Can you work these out from the model? Positions are in its coordinate system, mm. A direction names the side the tool comes from. Round coordinates to 2 decimals unless told otherwise and drop trailing zeros. Write each loop counter-clockwise with the first axis right and the second up, starting at its lowest first coordinate (ties: lowest second). Pieces come first, ordered by that corner, then holes. Notation, with made-up numbers: (44.5, 82.25) - (103.5, 82.25) arc R27 ccw to (103.5, 116.25) - close; hole circle Ø4 at (-33, 84.5). An arc over 180 degrees is marked (long way). One line per item, written item: value. Start each with the question number.
(1) On a 3-axis mill with a long thin cutter (end or side, diameter ignored), from which of +Z, -Z, +X, -X, +Y, -Y can I reach the whole of each face in a straight line? I mean faces 1 (the face through (3, 78.012, 3)), 2 (the face through (3, 135.162, 3)), 3 (the face through (168, 78.012, 3)). Say none if no direction works.
(2) I want a section at A-A on z = 2. Give the number of separate pieces and of enclosed holes in the cut face, plus the area to 3 significant figures.
(3) I want a section at C-C on y = 71. List the corners of the cut face in (x, z) for me, plus the area to 3 significant figures.
(4) If I drill on L1, parallel to X at y = 128.5, z = 1.5; L2, parallel to X at y = 117.5, z = 1; L3, parallel to Y at x = 203, z = 2, over which ranges is the centre line in solid material (lowest first)? Write a range as from..to.
(5) I want a section at B-B on x = 142. List the corners of the cut face in (y, z) for me, plus the area to 3 significant figures.
(6) I'm going to push flat-ended pins straight in: pin 1 Ø1.5 at (x, z) = (180.5, 2) entering from -Y; pin 2 Ø3 at (x, z) = (6.5, 3) entering from +Y. Where does each tip first touch, or does it pass through?
Autodesk Inventor part; units mm, degrees
ref_plane "YZ Plane" through (0, 0, 0) normal (1, 0, 0) x (0, 1, 0)
ref_plane "XZ Plane" through (0, 0, 0) normal (0, 1, 0) x (-1, 0, 0)
ref_plane "XY Plane" through (0, 0, 0) normal (0, 0, 1) x (1, 0, 0)
sketch "Sketch1" plane through (0, 0, 0) normal (0, 0, 1) x (1, 0, 0)
  line L0 (0, 78.0122) -> (0, 82.508)
  line L1 (-6.35, 82.508) -> (-6.35, 78.0122)
  line L2 (-6.35, 78.0122) -> (0, 78.0122)
  line L3 (222.25, 130.6664) -> (222.25, 135.1622)
  line L4 (215.9, 135.1622) -> (222.25, 135.1622)
  line L5 (215.9, 135.1622) -> (215.9, 130.6664)
  line L6 (222.25, 78.0122) -> (222.25, 135.1622)
  line L7 (-6.35, 135.1622) -> (-6.35, 78.0122)
  arc A0 (65.1726, 108.6235) -> (63.7223, 104.0872) centre (63.7223, 106.5872) ccw
  line L8 (222.25, 135.1622) -> (108.3945, 135.1622)
  line L9 (19.05, 135.1622) -> (-6.35, 135.1622)
  line L10 (-6.35, 78.0122) -> (19.05, 78.0122)
  line L11 (108.3945, 78.0122) -> (222.25, 78.0122)
  arc A1 (108.3945, 135.1622) -> (19.05, 135.1622) centre (63.7223, 106.5872) ccw
  arc A2 (19.05, 78.0122) -> (108.3945, 78.0122) centre (63.7223, 106.5872) ccw
  line L12 (215.9, 130.6664) -> (222.25, 130.6664)
  line L13 (0, 82.508) -> (-6.35, 82.508)
  point P0 (0, 0)
  dimension "d19" = 57.15
  dimension "d20" = 57.15
  dimension "d21" = 228.6
  dimension "d22" = 228.6
  dimension "d23" = 25.4
  dimension "d24" = 25.4
  dimension "d25" = 113.8555
  dimension "d26" = 113.8555
extrude "Extrusion1" add sketch "Sketch1" along normal blind 6.35
extrude "Extrusion2" [suppressed]
sketch "Sketch3" plane through (0, 0, 0) normal (0, 0, -1) x (-1, 0, 0)
  line L0 (6.35, 135.1622) -> (6.35, 78.0122) construction
  line L1 (-222.25, 135.1622) -> (-108.3945, 135.1622) construction
  line L2 (-222.25, 78.0122) -> (-222.25, 135.1622) construction
  line L3 (-108.3945, 78.0122) -> (-222.25, 78.0122) construction
  line L4 (-215.9, 135.1622) -> (-215.9, 130.6664) construction
  line L5 (-217.6131, 96.5879) -> (-200.4173, 96.5879) construction
  line L6 (-200.4173, 90.2379) -> (-217.6131, 90.2379) construction
  line L7 (-217.6131, 90.2379) -> (-217.6131, 96.5879) construction
  line L8 (-217.6131, 121.9879) -> (-200.4173, 121.9879) construction
  line L9 (-200.4173, 115.6379) -> (-217.6131, 115.6379) construction
  line L10 (-217.6131, 115.6379) -> (-217.6131, 121.9879) construction
  circle A0 centre (-219.075, 128.8122) radius 1.8542
  circle A1 centre (-198.5631, 118.6522) radius 1.8542
  line L11 (-222.25, 106.5872) -> (-215.9, 106.5872) construction
  circle A2 centre (-219.075, 84.3622) radius 1.8542
  circle A3 centre (-198.5631, 94.5222) radius 1.8542
  line L12 (-107.95, 135.1622) -> (-107.95, 78.0122) construction
  circle A4 centre (3.175, 128.8122) radius 1.8542
  circle A5 centre (-17.3369, 118.6522) radius 1.8542
  circle A6 centre (-17.3369, 94.5222) radius 1.8542
  circle A7 centre (3.175, 84.3622) radius 1.8542
  line L13 (-200.4173, 121.9879) -> (-200.4173, 115.6379)
  line L14 (-200.4173, 96.5879) -> (-200.4173, 90.2379)
  line L15 (6.35, 78.0122) -> (-19.05, 78.0122)
  line L16 (-19.05, 135.1622) -> (6.35, 135.1622)
  point P0 (0, 0)
  point P1 (-215.9, 135.1622)
  dimension "d7" = 3.7084
  dimension "d8" = 3.175
  dimension "d9" = 3.175
  dimension "d10" = 6.35
  dimension "d11" = 3.7084
  dimension "d12" = 19.05
  dimension "d13" = 28.575
  dimension "d14" = 28.575
  dimension "d15" = 114.3
  dimension "d16" = 114.3
  dimension "d27" = 16.51
  dimension "d28" = 16.51
  dimension "d29" = 23.6868
  dimension "d30" = 23.6868
  dimension "d31" = 16.51
  dimension "d32" = 16.51
  dimension "d33" = 23.6868
  dimension "d34" = 23.6868
extrude "Extrusion3" cut sketch "Sketch3" against normal through all
sketch "Sketch4" plane through (0, 0, 6.35) normal (0, 0, 1) x (1, 0, 0)
  line L0 (222.25, 135.1622) -> (228.6, 135.1622)
  line L1 (228.6, 135.1622) -> (228.6, 78.0122)
  line L2 (228.6, 78.0122) -> (222.25, 78.0122)
  line L3 (222.25, 78.0122) -> (222.25, 135.1622)
  line L4 (-6.35, 78.0122) -> (-12.7, 78.0122)
  line L5 (-12.7, 78.0122) -> (-12.7, 135.1622)
  line L6 (-12.7, 135.1622) -> (-6.35, 135.1622)
  line L7 (-6.35, 135.1622) -> (-6.35, 78.0122)
  point P0 (0, 0)
  dimension "d35" = 6.35
  dimension "d36" = 57.15
  dimension "d37" = 6.35
  dimension "d38" = 57.15
extrude "Extrusion4" add sketch "Sketch4" against normal blind 6.35
sketch "Sketch5" plane through (0, 0, 6.35) normal (0, 0, 1) x (1, 0, 0)
  line L0 (228.6, 135.1622) -> (228.6, 78.0122)
  line L1 (-12.7, 78.0122) -> (-12.7, 135.1622)
  line L2 (255.1581, 125.1613) -> (255.1581, 88.0132)
  line L3 (261.5081, 88.0132) -> (255.1581, 88.0132)
  line L4 (261.5081, 88.0132) -> (261.5081, 125.1613)
  line L5 (261.5081, 125.1613) -> (255.1581, 125.1613)
  line L6 (-6.35, 125.1613) -> (-6.35, 88.0132)
  line L7 (0, 88.0132) -> (-6.35, 88.0132)
  line L8 (0, 88.0132) -> (0, 125.1613)
  line L9 (0, 125.1613) -> (-6.35, 125.1613)
  line L10 (255.1581, 119.2872) -> (261.5081, 119.2872)
  line L11 (261.5081, 119.2872) -> (261.5081, 93.8872)
  line L12 (261.5081, 93.8872) -> (255.1581, 93.8872)
  line L13 (255.1581, 93.8872) -> (255.1581, 119.2872)
  line L14 (-12.7, 106.5872) -> (228.6, 106.5872) construction
  line L15 (107.95, 135.1622) -> (107.95, 78.0122) construction
  line L16 (-6.35, 125.1613) -> (0, 125.1613)
  line L17 (-39.2581, 119.2872) -> (-45.6081, 119.2872)
  line L18 (-45.6081, 119.2872) -> (-45.6081, 93.8872)
  line L19 (-45.6081, 93.8872) -> (-39.2581, 93.8872)
  line L20 (-39.2581, 93.8872) -> (-39.2581, 119.2872)
  point P0 (0, 0)
  dimension "d41" = 25.4
  dimension "d43" = 5.874
  dimension "d44" = 5.874
  dimension "d45" = 120.65
  dimension "d46" = 120.65
extrude "Extrusion5" cut sketch "Sketch5" against normal through all contours L10 L4 L12 L2 | L20 L19 L18 L17
sketch "Sketch6" plane through (0, 0, 6.35) normal (0, 0, 1) x (1, 0, 0)
  circle A0 centre (95.3576, 24.463) radius 3.175 construction
  circle A1 centre (97.1959, 37.4808) radius 1.8542
  circle A2 centre (108.3755, 22.6247) radius 1.8542
  circle A3 centre (93.5193, 11.4451) radius 1.8542
  circle A4 centre (82.3397, 26.3012) radius 1.8542
  circle A5 centre (95.3576, 24.463) radius 19.05 construction
  point P0 (0, 0)
extrude "Extrusion6" cut sketch "Sketch6" against normal through all
equation "\"d8\" = d9"
equation "\"d13\" = d14"
equation "\"d15\" = d16"
equation "\"d43\" = d44"
equation "\"d45\" = d46"
properties part number "tiltStructureCrossBeamRB01" material "Wood (Cherry)"
Established:
1. face 1: +Z, -Z, -X, -Y
1. face 2: +Z, -Z, -X, +Y
1. face 3: +Z, -Z, +X, -Y
2. separate pieces: 1
2. enclosed holes: 8
2. area: 16,800 mm2
3. outline: (24.41, 0) - (103.04, 0) - (103.04, 6.35) - (24.41, 6.35) - close
3. area: 499 mm2
4. L1: -12.7..-5, -1.35..217.25, 220.9..228.6
4. L2: -12.7..15.88, 18.79..197.11, 200.02..228.6
4. L3: 78.01..135.16
5. outline: (78.01, 0) - (135.16, 0) - (135.16, 6.35) - (78.01, 6.35) - close
5. area: 363 mm2
6. pin 1: y = 78.01
6. pin 2: y = 135.16
